```python
from build123d import *

# Parameters (mm, degrees)
SKETCH1_R           = 18.161
BOSS_EXTRUDE1_DEPTH = 17.653
SKETCH2_R           = 16.51
BOSS_EXTRUDE2_DEPTH = 22.606
SKETCH3_R           = 4.5085
BOSS_EXTRUDE3_DEPTH = 3.302
SKETCH4_R           = 2.413
BOSS_EXTRUDE4_DEPTH = 1.27
SKETCH5_R           = 5.969
BOSS_EXTRUDE5_DEPTH = 4.3688
BOSS_EXTRUDE6_DEPTH = 15.24
SKETCH8_W           = 5.588
SKETCH8_H           = 2.794
SKETCH8_R           = 0.635
BOSS_EXTRUDE7_DEPTH = 0.254
CIRPATTERN1_COUNT   = 2
CIRPATTERN2_COUNT   = 12


with BuildPart() as part:
    # Sketch1 → Boss-Extrude1 (new body)
    with BuildSketch(Plane.XY):
        Circle(SKETCH1_R)
    extrude(amount=BOSS_EXTRUDE1_DEPTH)

    # Sketch2 → Boss-Extrude2 (add)
    with BuildSketch(Plane(origin=(0, 0, 0), x_dir=(-1, 0, 0), z_dir=(0, 0, -1))):
        Circle(SKETCH2_R)
    extrude(amount=BOSS_EXTRUDE2_DEPTH)

    # Sketch3 → Boss-Extrude3 (add)
    with BuildSketch(Plane(origin=(0, 0, -22.606), x_dir=(-1, 0, 0), z_dir=(0, 0, -1))):
        Circle(SKETCH3_R)
    extrude(amount=BOSS_EXTRUDE3_DEPTH)

    # Sketch4 → Boss-Extrude4 (add)
    with BuildSketch(Plane(origin=(0, 0, -22.606), x_dir=(-1, 0, 0), z_dir=(0, 0, -1))):
        with Locations((0, -12.7)):
            Circle(SKETCH4_R)
        with Locations((0, 12.7)):
            Circle(SKETCH4_R)
    extrude(amount=BOSS_EXTRUDE4_DEPTH)

    # Sketch5 → Boss-Extrude5 (add)
    with BuildSketch(Plane.XY.offset(17.653)):
        with Locations((0, -7.366)):
            Circle(SKETCH5_R)
    extrude(amount=BOSS_EXTRUDE5_DEPTH)

    # Sketch6 → Boss-Extrude6 (add)
    with BuildSketch(Plane.XY.offset(22.0218)):
        with BuildLine():
            Line((-1.715657017, -4.905), (1.715657017, -4.905))
            ThreePointArc((1.715657017, -4.905), (0, -10.366), (-1.715657017, -4.905))
        make_face()
    extrude(amount=BOSS_EXTRUDE6_DEPTH)

    # Sketch8 → Boss-Extrude7 (add, symmetric)
    with BuildSketch(Plane.ZX.offset(12.7)):
        with Locations((-26.67, 0)):
            Rectangle(SKETCH8_W, SKETCH8_H)
        with Locations((-28.067, 0)):
            Circle(SKETCH8_R, mode=Mode.SUBTRACT)
    boss_extrude7 = extrude(amount=BOSS_EXTRUDE7_DEPTH, both=True)

    # CirPattern1: Boss-Extrude7 ×2 about axis
    cirpattern1_axis = Axis((0, 0, 0), (0, 0, 1))
    for i in range(1, CIRPATTERN1_COUNT):
        add(boss_extrude7.rotate(cirpattern1_axis, i * 360 / CIRPATTERN1_COUNT))

    # Sketch12 → 3.0mm Dowel Hole1 (revolve, cut)
    with BuildSketch(Plane(origin=(0, 15.494, 17.653), x_dir=(0, -1, 0), z_dir=(1, 0, 0))):
        Polygon((0, 0), (0, 11.061290929), (1.5, 10.16), (1.5, 0), align=None)
    f_3_0mm_dowel_hole1 = revolve(axis=Axis((0, 15.494, 24.003), (0, 0, -1)), mode=Mode.SUBTRACT)

    # CirPattern2: 3.0mm Dowel Hole1 ×12 about axis, 5 skipped
    cirpattern2_axis = Axis((0, 0, 17.653), (0, 0, -1))
    add([f_3_0mm_dowel_hole1.rotate(cirpattern2_axis, i * 360 / CIRPATTERN2_COUNT) for i in range(1, CIRPATTERN2_COUNT) if i not in (1, 2, 5, 6, 10)], mode=Mode.SUBTRACT)


solid = part.part
```
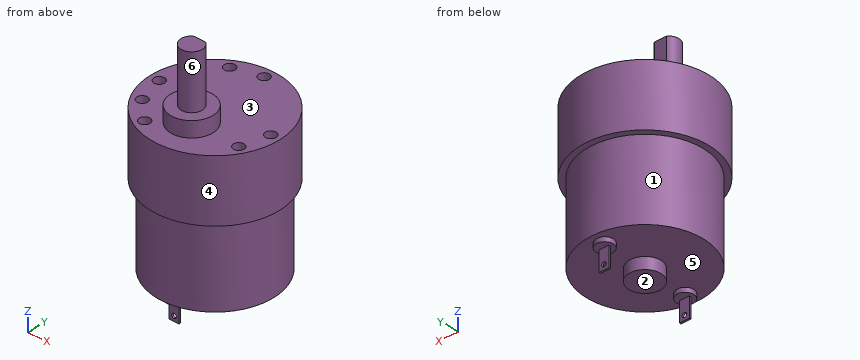
Geometry check sheet. Reference: the model listing, model coordinates, mm. Face numbers are marked on the shaded views. A direction names the side the tool comes from. Give positions to 0.01 mm unless a question says otherwise; leave off trailing zeros. Write each loop counter-clockwise with the first axis right and the second up, starting at its lowest first coordinate (ties: lowest second). Pieces come first, ordered by that corner, then holes.
1) Material ranges on L1, parallel to Y at x = 0, z = -13.5; L2, parallel to Z at x = 0, y = 12; L3, parallel to Z at x = 0, y = -12.7, recorded low to high.
2) Section check B-B, the plane z = -10. Record the boundary of the cut face in (x, y), and give its area (3 significant figures).
3) Access from +Z, -Z, +X, -X, +Y, -Y to the whole of each face (thin tool, end or side, straight path). Record for the marked faces 4, 5 and 6.
4) Release check for a two-part mould opening along Y. For the marked faces 1, 2 and 3 record: pulls with the +Y half, pulls with the -Y half, needs draft (parallel to the pull), parting line crosses it, or undercut.
5) Section check A-A, the plane y = 5.5. Record the boundary of the cut face in (x, z), and give its area (3 significant figures).
6) Gauge pin test, flat ends, axial feed: pin 1 (1.5 mm diameter, centred on y = -11, z = -20, fed in from +X); pin 2 (1.8 mm diameter, centred on x = 15.494, y = 0, fed in from -Z); pin 3 (6 mm diameter, centred on y = -5.5, z = 11, fed in from +X); pin 4 (4 mm diameter, centred on y = 1.5, z = 2, fed in from +X). Record the tip position at first contact, or that the pin passes through.
7) Section check C-C, the plane z = 21. Record the boundary of the cut face in (x, y), and give its area (3 significant figures).
Computed:
1. L1: y = -16.51 to 16.51
1. L2: z = -23.88 to 17.65
1. L3: z = -29.46 to -28.7, -27.43 to 22.02
2. outline: circle Ø33.02 at (0, 0)
2. area: 856 mm2
3. face 4: +Z, -Z
3. face 5: -Z
3. face 6: +Z
4. face 1: parting line crosses it
4. face 2: undercut
4. face 3: needs draft
5. outline: (-17.31, 0) - (-15.57, 0) - (-15.57, -22.61) - (15.57, -22.61) - (15.57, 0) - (17.31, 0) - (17.31, 17.65) - (-17.31, 17.65) - close
5. area: 1,310 mm2
6. pin 1: stops at x = 12.94
6. pin 2: stops at z = -22.61
6. pin 3: stops at x = 17.99
6. pin 4: stops at x = 18.16
7. outline: circle Ø11.94 at (0, -7.37)
7. area: 112 mm2
